from build123d import *

# Parameters (mm, degrees)
BOSS_EXTRUDE1_DEPTH = 5.55625
BOSS_EXTRUDE2_DEPTH = 1.5875
SKETCH6_R           = 1.5875
BOSS_EXTRUDE3_DEPTH = 5.55625


with BuildPart() as part:
    # Sketch1 → Boss-Extrude1 (new body, symmetric)
    with BuildSketch(Plane(origin=(0, 0, 0), x_dir=(0, 0, -1), z_dir=(1, 0, 0))):
        with BuildLine():
            ThreePointArc((-6.261184437, 17.991666667), (0, -19.05), (6.261184437, 17.991666667))
            ThreePointArc((6.261184437, 17.991666667), (0, 12.7), (-6.261184437, 17.991666667))
        make_face()
        with BuildLine():
            ThreePointArc((-7.919841469, 13.758333333), (0, 9.525), (7.919841469, 13.758333333))
            ThreePointArc((7.919841469, 13.758333333), (0, -15.875), (-7.919841469, 13.758333333))
        make_face(mode=Mode.SUBTRACT)
    extrude(amount=BOSS_EXTRUDE1_DEPTH, both=True)

    # Sketch3 → Boss-Extrude2 (add, symmetric)
    with BuildSketch(Plane(origin=(0, 0, 0), x_dir=(0, 0, -1), z_dir=(1, 0, 0))):
        with BuildLine():
            ThreePointArc((-7.919841469, 13.758333333), (0, -15.875), (7.919841469, 13.758333333))
            ThreePointArc((7.919841469, 13.758333333), (0, 9.525), (-7.919841469, 13.758333333))
        make_face()
    extrude(amount=BOSS_EXTRUDE2_DEPTH, both=True)

    # Sketch6 → Boss-Extrude3 (add, symmetric)
    with BuildSketch(Plane(origin=(0, 0, 0), x_dir=(0, 0, -1), z_dir=(1, 0, 0))):
        Circle(SKETCH6_R)
    extrude(amount=BOSS_EXTRUDE3_DEPTH, both=True)


solid = part.part
Read the model definition and answer for the solid it produces. Units are mm, in the model's axes. A direction names the side the tool comes from. Give positions to 0.01 mm unless a question says otherwise; leave off trailing zeros. Write each loop counter-clockwise with the first axis right and the second up, starting at its lowest first coordinate (ties: lowest second). Pieces come first, ordered by that corner, then holes. Notation, with made-up numbers: (-8, 26.25) - (49, 26.25) arc R14 cw to (49, 43.25) - close; hole circle Ø6 at (43.25, 62.5). An arc over 180 degrees is marked (long way). Use CSV: the item, a comma, the result in double quotes. Start each with the question number.
(1) Determine the mould class of faces 4 (the flat face through (-5.556, 0, 0)), 5 (the cylindrical face through (3.6, 9.526, 0.131)), 6 (the cylindrical face through (-3.544, -15.864, -0.582)), 7 (the cylindrical face through (0.078, -19.035, 0.748)) for opening direction Y: +Y half, -Y half, draft (parallel to the pull), parting line (faces both ways), or undercut.
(2) Consider line 1 along Z through (x, y) = (2, -1); line 2 along X through (y, z) = (-11, 9.5); line 3 along Z through (x, y) = (-2.5, -6). Determine where each line is inside the solid, lowest interval first.
(3) Find section A-A (x = -2.5). Count the separate pieces of the cut face and the enclosed holes in it, plus the area to 3 significant figures.
(4) For faces 1 (the cylindrical face through (3.6, -1.55, 0.34)), 2 (the flat face through (-5.556, 11, 2)), 3 (the flat face through (-1.588, -4, 0)), determine the directions among +Z, -Z, +X, -X, +Y, -Y from which every point of the face is accessible in a straight line to the end or side of a thin tool.
(5) Given P1, Ø3, axis at x = -4, y = 9.5, coming from the -Z side; P2, Ø9, axis at y = 6, z = 1, coming from the +X side; P3, Ø2, axis at y = 3.5, z = 2.5, coming from the +X side; P4, Ø6, axis at x = -2, z = 5, coming from the +Y side, each flat-ended and moving along its own axis, determine where each tip first touches the part or whether it passes through.
(6) Find section D-D (x = 0.5). Give the vertices of the cut face in (y, z), plus the area to 3 significant figures.
Findings below:
1,face 4,"draft"
1,face 5,"undercut"
1,face 6,"undercut"
1,face 7,"parting line"
2,line 1,"-19.02 to -15.84, -1.23 to 1.23, 15.84 to 19.02"
2,line 2,"-1.59 to 1.59"
2,line 3,"-18.08 to -14.7, 14.7 to 18.08"
3,separate pieces,"2"
3,enclosed holes,"1"
3,area,"367 mm2"
4,face 1,"+X"
4,face 2,"+Z, -Z, -X, +Y, -Y"
4,face 3,"-X"
5,P1,"z = -17.29"
5,P2,"x = 5.56"
5,P3,"x = 1.59"
5,P4,"y = 17.99"
6,outline,"(17.99, -6.26) arc R6.35 cw to (17.99, 6.26) arc R19.05 ccw (long way) to start"
6,area,"1,080 mm2"
